The listing builds one solid part. Answer for the finished solid, in the listing's coordinates (mm). Give positions to 0.01 mm unless a question says otherwise; leave off trailing zeros. Order: outer loops, then holes, each group sorted by start corner. A loop starts at its lowest first (then second) coordinate and runs counter-clockwise, first axis right, second up. Notation, with made-up numbers: (-19, -4) - (-11, -4) arc R15 ccw to (-11, 20) - close; hole circle Ø7 at (-32.5, 46). An arc over 180 degrees is marked (long way). Use a Markdown table: item, result. Add a question column.
1) Find section D-D, the plane z = 1.2. State how many separate pieces and enclosed holes the cut face has, plus the area to 3 significant figures.
2) Find section A-A, the plane y = -12.5. Determine the outline of the cut face in (x, z).
3) Find section C-C, the plane y = 22. Determine the outline of the cut face in (x, z), plus the area to 3 significant figures.
4) Flat-ended cylindrical pins translate along their axes: pin 1 (1.5 mm diameter, centred on x = 23, z = 1.5, fed in from -Y); pin 2 (1 mm diameter, centred on x = -17, z = 2.5, fed in from +Y); pin 3 (1.5 mm diameter, centred on x = 78.5, z = 1.5, fed in from -Y). Find the tip coordinate at first contact, or state that the pin passes through.
5) Find section B-B, the plane x = 90. Determine the outline of the cut face in (y, z), plus the area to 3 significant figures.
6) Straight lines are drawn through the part: line 1 (Y direction, x = -3, z = 2.1); line 2 (Y direction, x = 48, z = 0.9); line 3 (X direction, y = 27.5, z = 2.65). For each, find the intervals that lie inside material, in ascending order.
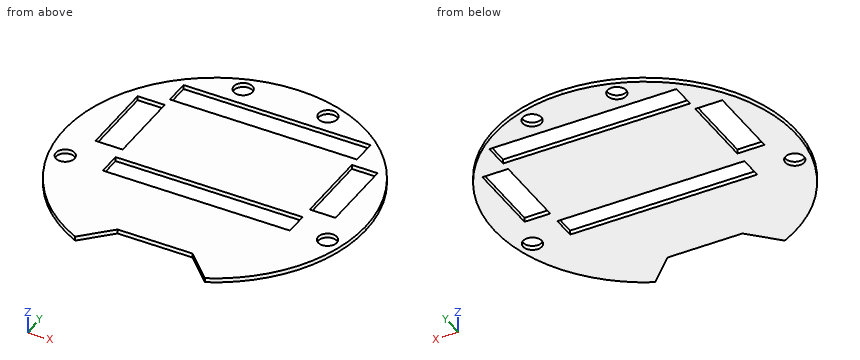
from build123d import *

# Parameters (mm, degrees)
F0_R     = 6.5
F0_W     = 18.890693
F0_H     = 53.3
F0_W_2   = 17.913587
F1_DEPTH = 3


with BuildPart() as f1:
    # F0 (on Top) → F1 (new body)
    with BuildSketch(Plane.XY):
        with BuildLine():
            Line((-0.027255, 77.031374), (-0.027255, 106.016069))
            ThreePointArc((-0.027255, 106.016069), (-102.446612, 24.152087), (-45.162038, -93.788211))
            Line((-45.162038, -93.788211), (-26.15007, -74.776243))
            Line((-26.15007, -74.776243), (-0.027255, -74.776243))
            Line((-0.027255, -74.776243), (-0.027255, -63.699956))
            Line((-0.027255, -63.699956), (-0.027255, -48.653428))
            Line((-0.027255, -48.653428), (-0.027255, -25.119923))
            Line((-0.027255, -25.119923), (-63.711368, -25.119923))
            Line((-63.711368, -25.119923), (-63.711368, -8.998516))
            Line((-63.711368, -8.998516), (-0.027255, -8.998516))
            Line((-0.027255, -8.998516), (-0.027255, 0))
            Line((-0.027255, 0), (-50.827254, 0))
            Line((-50.827254, 0), (-50.827254, 53.3))
            Line((-50.827254, 53.3), (-0.027255, 53.3))
            Line((-0.027255, 53.3), (-0.027255, 59.769183))
            Line((-0.027255, 59.769183), (-63.711368, 59.769183))
            Line((-63.711368, 59.769183), (-63.711368, 77.031374))
            Line((-63.711368, 77.031374), (-0.027255, 77.031374))
        make_face()
        with Locations((-91.341169, -22.449345)):
            Circle(F0_R, mode=Mode.SUBTRACT)
        with Locations((-73.156714, 26.65)):
            Rectangle(F0_W, F0_H, mode=Mode.SUBTRACT)
        with Locations((-29.749685, 90.793084)):
            Circle(F0_R, mode=Mode.SUBTRACT)
        with BuildLine():
            ThreePointArc((45.107527, -93.788211), (88.753802, -55.045718), (104.972745, 1.016069))
            ThreePointArc((104.972745, 1.016069), (74.218957, 75.262281), (-0.027255, 106.016069))
            Line((-0.027255, 106.016069), (-0.027255, 77.031374))
            Line((-0.027255, 77.031374), (66.569284, 77.031374))
            Line((66.569284, 77.031374), (66.569284, 59.769183))
            Line((66.569284, 59.769183), (-0.027255, 59.769183))
            Line((-0.027255, 59.769183), (-0.027255, 53.3))
            Line((-0.027255, 53.3), (50.772746, 53.3))
            Line((50.772746, 53.3), (50.772746, 0))
            Line((50.772746, 0), (-0.027255, 0))
            Line((-0.027255, 0), (-0.027255, -8.998516))
            Line((-0.027255, -8.998516), (66.569284, -8.998516))
            Line((66.569284, -8.998516), (66.569284, -25.119923))
            Line((66.569284, -25.119923), (-0.027255, -25.119923))
            Line((-0.027255, -25.119923), (-0.027255, -48.653428))
            Line((-0.027255, -48.653428), (-0.027255, -63.699956))
            Line((-0.027255, -63.699956), (-0.027255, -74.776243))
            Line((-0.027255, -74.776243), (26.095559, -74.776243))
            Line((26.095559, -74.776243), (45.107527, -93.788211))
        make_face()
        with Locations((91.286659, -22.449345)):
            Circle(F0_R, mode=Mode.SUBTRACT)
        with Locations((75.526077, 26.65)):
            Rectangle(F0_W_2, F0_H, mode=Mode.SUBTRACT)
        with Locations((29.269962, 90.793084)):
            Circle(F0_R, mode=Mode.SUBTRACT)
        Polygon((50.772746, 53.3), (-0.027255, 53.3), (-0.027255, 1.016069), (-0.027255, 0), (50.772746, 0), align=None)
        Polygon((-0.027255, 1.016069), (-0.027255, 53.3), (-50.827254, 53.3), (-50.827254, 0), (-0.027255, 0), align=None)
    extrude(amount=F1_DEPTH)


solid = f1.part
The answers:
| question | item | result |
|---|---|---|
| 1 | separate pieces | 1 |
| 1 | enclosed holes | 8 |
| 1 | area | 25,800 mm2 |
| 2 | outline | (-104.15, 0) - (-63.71, 0) - (-63.71, 3) - (-104.15, 3) - close; (66.57, 0) - (104.1, 0) - (104.1, 3) - (66.57, 3) - close |
| 3 | outline | (-102.91, 0) - (-82.6, 0) - (-82.6, 3) - (-102.91, 3) - close; (-63.71, 0) - (66.57, 0) - (66.57, 3) - (-63.71, 3) - close; (84.48, 0) - (102.85, 0) - (102.85, 3) - (84.48, 3) - close |
| 3 | area | 507 mm2 |
| 4 | pin 1 | y = -74.78 |
| 4 | pin 2 | y = 104.72 |
| 4 | pin 3 | y = -69.52 |
| 5 | outline | (-53.02, 0) - (-28.82, 0) - (-28.82, 3) - (-53.02, 3) - close; (-16.08, 0) - (55.05, 0) - (55.05, 3) - (-16.08, 3) - close |
| 5 | area | 286 mm2 |
| 6 | line 1 | -74.78 to -25.12, -9 to 59.77, 77.03 to 105.97 |
| 6 | line 2 | -92.36 to -25.12, -9 to 59.77, 77.03 to 94.39 |
| 6 | line 3 | -101.63 to -82.6, -63.71 to 66.57, 84.48 to 101.58 |
